Here's how the part is built. I have some questions about the finished solid (model axes, mm). A direction names the side the tool comes from. Round coordinates to 2 decimals unless told otherwise and drop trailing zeros. Write each loop counter-clockwise with the first axis right and the second up, starting at its lowest first coordinate (ties: lowest second). Pieces come first, ordered by that corner, then holes. Notation, with made-up numbers: (66.25, -5.5) -> (101.25, -5.5) arc R15 cw to (101.25, 15.5) -> close; hole circle Ø1 at (32, 27.5). An arc over 180 degrees is marked (long way). Answer as CSV lines item,"result".
from build123d import *

# Parameters (mm, degrees)
SKETCH1_R           = 1.5875
BOSS_EXTRUDE1_DEPTH = 1.6002
CHAMFER1_SIZE       = 0.762


with BuildPart() as part:
    # Sketch1 → Boss-Extrude1 (new body)
    with BuildSketch(Plane(origin=(0, 0, 0), x_dir=(1, 0, 0), z_dir=(0, 1, 0))):
        Polygon((0, 0), (0, 53.34), (67.31, 53.34), (67.31, 40.64), (71.12, 36.83), (71.12, 6.35), (67.31, 2.54), (67.31, 0), align=None)
        with Locations(Location((16.51, 50.8, 0), (0, 0, 270))):
            Circle(SKETCH1_R, mode=Mode.SUBTRACT)
        with Locations(Location((15.24, 2.54, 0), (0, 0, 270))):
            Circle(SKETCH1_R, mode=Mode.SUBTRACT)
        with Locations(Location((67.31, 35.56, 0), (0, 0, 270))):
            Circle(SKETCH1_R, mode=Mode.SUBTRACT)
        with Locations(Location((67.31, 7.62, 0), (0, 0, 270))):
            Circle(SKETCH1_R, mode=Mode.SUBTRACT)
    extrude(amount=BOSS_EXTRUDE1_DEPTH)

    # Chamfer1
    chamfer1_edges = [part.edges().sort_by_distance(p)[0] for p in [
        (0, 0.8001, 0),
        (0, 0.8001, -53.34),
        (67.31, 0.8001, -53.34),
        (67.31, 0.8001, 0),
    ]]
    chamfer(chamfer1_edges, length=CHAMFER1_SIZE)


solid = part.part
Item 1: If we mould it in two halves opening along Z, with no side actions, what happens to faces 4 (the flat face through (69.19, 0.79, -38.76)), 5 (the flat face through (69.24, 0.79, -4.47)), 6 (the cylindrical face through (68.884, 0.789, -35.767))? For each: pulls with the +Z half, pulls with the -Z half, needs draft (parallel to the pull), parting line crosses it, or undercut.
Results found:
face 4,"pulls with the -Z half"
face 5,"pulls with the +Z half"
face 6,"undercut"
Item 2: Suppose I cut it at A-A, the plane z = -7.62. List the corners of the cut face in (x, y) for me.
Results found:
outline,"(0, 0) -> (65.72, 0) -> (65.72, 1.6) -> (0, 1.6) -> close; (68.9, 0) -> (71.12, 0) -> (71.12, 1.6) -> (68.9, 1.6) -> close"
Item 3: Suppose I cut it at B-B, the plane y = 0.75. State how many separate pieces and enclosed holes the cut face has, then the cut area to 3 significant figures.
Results found:
separate pieces,"1"
enclosed holes,"4"
area,"3,690 mm²"
Item 4: Suppose I cut it at C-C, the plane z = -50.8. List the corners of the cut face in (x, y) for me, then the cut area to 3 significant figures.
Results found:
outline,"(0, 0) -> (14.92, 0) -> (14.92, 1.6) -> (0, 1.6) -> close; (18.1, 0) -> (67.31, 0) -> (67.31, 1.6) -> (18.1, 1.6) -> close"
area,"103 mm²"
Item 5: For faces 1 (the flat face through (67.31, 1, -47)), 2 (the flat face through (33, 1, -53.34)), 3 (the flat face through (67.31, 1, -2)), which set-ups out of +Z, -Z, +X, -X, +Y, -Y let a thin tool reach every point of the face, with its end or its side?
Results found:
face 1,"-Z, +X, +Y, -Y"
face 2,"-Z, +X, -X, +Y, -Y"
face 3,"+Z, +X, +Y, -Y"
Item 6: I need wall thicknesses on L1, parallel to X at y = 0.75, z = -35.56; L2, parallel to X at y = 0.85, z = -50.8; L3, parallel to X at y = 1.55, z = -42.5. Which ranges of each line are inside material? Lowest first, please.
Results found:
L1,"x = 0 to 65.72, 68.9 to 71.12"
L2,"x = 0 to 14.92, 18.1 to 67.31"
L3,"x = 0 to 67.31"
